```python
from build123d import *

# Parameters (mm, degrees)
SKETCH1_W           = 20
SKETCH1_H           = 48
SKETCH1_W_2         = 8
BOSS_EXTRUDE1_DEPTH = 6
SKETCH1_3_W         = 20
SKETCH1_3_H         = 48
BOSS_EXTRUDE2_DEPTH = 14
SKETCH2_R           = 0.875
CUT_EXTRUDE1_DEPTH  = 25
SKETCH3_R           = 1.25
CUT_EXTRUDE2_DEPTH  = 25


with BuildPart() as part:
    # Sketch1 → Boss-Extrude1 (new body)
    with BuildSketch(Plane.XY):
        with Locations((-14, 0)):
            Rectangle(SKETCH1_W, SKETCH1_H)
        Rectangle(SKETCH1_W_2, SKETCH1_H)
        with Locations((14, 0)):
            Rectangle(SKETCH1_W, SKETCH1_H)
    extrude(amount=BOSS_EXTRUDE1_DEPTH)

    # Sketch1_3 → Boss-Extrude2 (add)
    with BuildSketch(Plane.XY):
        with Locations((-14, 0)):
            Rectangle(SKETCH1_3_W, SKETCH1_3_H)
        with Locations((14, 0)):
            Rectangle(SKETCH1_3_W, SKETCH1_3_H)
    extrude(amount=BOSS_EXTRUDE2_DEPTH)

    # Sketch2 → Cut-Extrude1 (cut)
    with BuildSketch(Plane.ZY.offset(24)):
        with Locations((14, 0)):
            Circle(SKETCH2_R)
        with Locations((14, 10)):
            Circle(SKETCH2_R)
        with Locations((14, 20)):
            Circle(SKETCH2_R)
        with Locations((14, -10)):
            Circle(SKETCH2_R)
        with Locations((14, -20)):
            Circle(SKETCH2_R)
    extrude(amount=-CUT_EXTRUDE1_DEPTH, mode=Mode.SUBTRACT)

    # Sketch3 → Cut-Extrude2 (cut)
    with BuildSketch(Plane(origin=(24, 0, 0), x_dir=(0, 0, -1), z_dir=(1, 0, 0))):
        with Locations((-14, 0)):
            Circle(SKETCH3_R)
        with Locations((-14, -10)):
            Circle(SKETCH3_R)
        with Locations((-14, -20)):
            Circle(SKETCH3_R)
        with Locations((-14, 10)):
            Circle(SKETCH3_R)
        with Locations((-14, 20)):
            Circle(SKETCH3_R)
    extrude(amount=-CUT_EXTRUDE2_DEPTH, mode=Mode.SUBTRACT)


solid = part.part
```
CAD build for the part. Positions are in the model's coordinates, mm. A direction names the side the tool comes from. Round coordinates to 2 decimals unless told otherwise and drop trailing zeros. Order: outer loops, then holes, each group sorted by start corner. A loop starts at its lowest first (then second) coordinate and runs counter-clockwise, first axis right, second up. Notation, with made-up numbers: (-1.75, -7.75) - (25.25, -7.75) arc R9 cw to (25.25, 9.25) - close; hole circle Ø11 at (85.5, 81.5). An arc over 180 degrees is marked (long way). Answer as CSV lines item,"result". Start each with the question number.
1. Pin check, flat tips, straight feed: pin 1 (9 mm diameter, centred on x = 0.5, y = 2, fed in from +Z); pin 2 (5 mm diameter, centred on x = 0.5, y = -18.5, fed in from +Z). Stop position of each tip, or through.
2. Pull direction Y, two halves, no side cores. Call faces 1 (the face through (-24, 0, 7)), 2 (the face through (0, 24, 5)), 3 (the face through (14.14, -20.03, 12.75)): +Y half, -Y half, draft (parallel to the pull), parting line (faces both ways), or undercut.
3. Saw through at C-C, the plane x = 15. Write the cut outline in (y, z).
4. Drill centre lines: L1, parallel to X at y = 7, z = 12.5; L2, parallel to Z at x = 1.5, y = -16; L3, parallel to Z at x = 20.5, y = -20. Where is each one in solid material? Low to high. Write a range as [from, to].
5. Saw through at D-D, the plane x = 0.5. Write the cut outline in (y, z).
6. Saw through at B-B, the plane y = 0. Write the cut outline in (x, z) (3 decimals).
7. Saw through at A-A, the plane z = 6.75. Write the cut outline in (x, y), and give its area (3 significant figures).
8. Tool access for faces 4 (the face through (-4, 0, 10)), 5 (the face through (14.14, -10.03, 12.75)), 6 (the face through (24, 0, 7)): list every direction of +Z, -Z, +X, -X, +Y, -Y with a clear straight run to the whole face (end or side of a thin tool).
Model answer:
1,pin 1,"stops at z = 14"
1,pin 2,"stops at z = 6"
2,face 1,"draft"
2,face 2,"+Y half"
2,face 3,"undercut"
3,outline,"(-24, 0) - (24, 0) - (24, 14) - (21.25, 14) arc R1.25 cw to (18.75, 14) - (11.25, 14) arc R1.25 cw to (8.75, 14) - (1.25, 14) arc R1.25 cw to (-1.25, 14) - (-8.75, 14) arc R1.25 cw to (-11.25, 14) - (-18.75, 14) arc R1.25 cw to (-21.25, 14) - (-24, 14) - close"
4,L1,"x = [-24, -4], [4, 24]"
4,L2,"z = [0, 6]"
4,L3,"z = [0, 12.75]"
5,outline,"(-24, 0) - (24, 0) - (24, 6) - (-24, 6) - close"
6,outline,"(-24, 0) - (24, 0) - (24, 12.75) - (4, 12.75) - (4, 6) - (-4, 6) - (-4, 13.125) - (-24, 13.125) - close"
7,outline,"(-24, -24) - (-4, -24) - (-4, 24) - (-24, 24) - close; (4, -24) - (24, -24) - (24, 24) - (4, 24) - close"
7,area,"1,920 mm²"
8,face 4,"+Z, +Y, -Y"
8,face 5,"+Z, +X"
8,face 6,"+Z, -Z, +X, +Y, -Y"
